Build history of the part. All positions in model axes, mm. A direction names the side the tool comes from. Give positions to 0.01 mm unless a question says otherwise; leave off trailing zeros. Order: outer loops, then holes, each group sorted by start corner. A loop starts at its lowest first (then second) coordinate and runs counter-clockwise, first axis right, second up. Notation, with made-up numbers: (-32, 23) -> (2, 23) arc R25 cw to (2, 59) -> close; hole circle Ø7 at (3.5, 29). An arc over 180 degrees is marked (long way). One line per question, with ' | ' between items. Start each with the question number.
(1) Drill centre lines: L1, parallel to X at y = 57.15, z = 11; L2, parallel to Y at x = 24, z = 18; L3, parallel to X at y = 52, z = 18.5. Where is each one in solid material? Low to high. Write a range as from..to.
(2) Pull direction Z, two halves, no side cores. Call faces 1 (the face through (5.02, 55.83, 9.66)), 2 (the face through (52.37, 74.27, 15.73)), 3 (the face through (35, 39, 2.54)): +Z half, -Z half, draft (parallel to the pull), parting line (faces both ways), or undercut.
(3) Which spindle directions (+Z, -Z, +X, -X, +Y, -Y) get a long thin tool onto all of the face, cutting with end or side? Do faces 4 (the face through (64.41, 68.15, 10.68)), 5 (the face through (35, 76.2, 9)). Say none if no direction does.
(4) Pin check, flat tips, straight feed: pin 1 Ø10 at (x, y) = (41, 9.5) entering from +Z; pin 2 Ø2 at (x, y) = (64.77, 57.15) entering from -Z. Stop position of each tip, or through.
(5) Cut at A-A (y = 38.1). Give the cut face in (x, z), then the cut area to 3 significant figures.
(6) Cut at B-B (x = 16). Give the cut face in (y, z), then the cut area to 3 significant figures.
(7) Cut at C-C (y = 71). Give the cut face in (x, z), then the cut area to 3 significant figures.
Autodesk Inventor part; units mm, degrees
ref_plane "YZ Plane" through (0, 0, 0) normal (1, 0, 0) x (0, 1, 0)
ref_plane "XZ Plane" through (0, 0, 0) normal (0, 1, 0) x (-1, 0, 0)
ref_plane "XY Plane" through (0, 0, 0) normal (0, 0, 1) x (1, 0, 0)
sketch "Sketch1" plane through (0, 0, 0) normal (0, 0, 1) x (1, 0, 0)
  line L0 (0, 0) -> (69.85, 0)
  line L1 (69.85, 0) -> (69.85, 76.2)
  line L2 (69.85, 76.2) -> (0, 76.2)
  line L3 (0, 76.2) -> (0, 0)
  line L4 (0, 76.2) -> (7.62, 76.2)
  line L5 (7.62, 3.81) -> (62.23, 3.81)
  line L6 (58.42, 72.39) -> (7.62, 72.39)
  line L7 (7.62, 72.39) -> (11.43, 72.39)
  line L8 (0, 76.2) -> (69.85, 76.2)
  line L9 (34.925, 76.2) -> (50.165, 76.2)
  line L10 (50.165, 76.2) -> (50.165, 69.1676)
  line L11 (34.925, 76.2) -> (19.685, 76.2)
  line L12 (19.685, 76.2) -> (14.9225, 76.2)
  line L13 (0, 76.2) -> (0, 57.15)
  line L14 (19.685, 76.2) -> (13.9303, 76.2)
  arc A0 (11.43, 72.39) -> (7.62, 60.96) centre (11.43, 66.04) ccw
  line L15 (7.62, 3.81) -> (11.43, 3.81)
  line L16 (11.43, 3.81) -> (11.43, 10.16)
  line L17 (62.23, 3.81) -> (58.42, 3.81)
  line L18 (58.42, 3.81) -> (58.42, 10.16)
  arc A1 (7.62, 15.24) -> (11.43, 3.81) centre (11.43, 10.16) ccw
  arc A2 (58.42, 3.81) -> (62.23, 15.24) centre (58.42, 10.16) ccw
  arc A3 (62.23, 60.96) -> (58.42, 72.39) centre (58.42, 66.04) ccw
  line L19 (62.23, 15.24) -> (62.23, 60.96)
  line L20 (7.62, 60.96) -> (7.62, 15.24)
  dimension "d9" = 7.62
  dimension "d13" = 15.24
  dimension "d18" = 19.05
  dimension "d24" = 6.35
  dimension "d25" = 3.81
  dimension "d26" = 6.35
extrude "Extrusion1" add sketch "Sketch1" along normal blind 19.05
sketch "Sketch3" plane through (0, 0, 0) normal (0, 0, -1) x (-1, 0, 0)
  arc A0 (-11.43, 3.81) -> (-7.62, 15.24) centre (-11.43, 10.16) ccw
  line L0 (-11.43, 3.81) -> (-58.42, 3.81)
  arc A1 (-62.23, 15.24) -> (-58.42, 3.81) centre (-58.42, 10.16) ccw
  line L1 (-62.23, 15.24) -> (-62.23, 60.96)
  arc A2 (-58.42, 72.39) -> (-62.23, 60.96) centre (-58.42, 66.04) ccw
  line L2 (-58.42, 72.39) -> (-11.43, 72.39)
  arc A3 (-7.62, 60.96) -> (-11.43, 72.39) centre (-11.43, 66.04) ccw
  line L3 (-7.62, 60.96) -> (-7.62, 15.24)
  line L4 (0, 76.2) -> (0, 0)
  line L5 (-69.85, 76.2) -> (0, 76.2)
  line L6 (-69.85, 0) -> (-69.85, 76.2)
  line L7 (0, 0) -> (-69.85, 0)
  line L8 (0, 76.2) -> (-5.08, 76.2)
  line L9 (-69.85, 76.2) -> (0, 76.2)
  line L10 (-5.08, 76.2) -> (-5.08, 0)
  line L11 (-5.08, 76.2) -> (-5.08, 57.15)
  line L12 (-5.08, 0) -> (-5.08, 19.05)
  line L13 (-69.85, 0) -> (-64.77, 0)
  line L14 (0, 0) -> (-69.85, 0)
  line L15 (-64.77, 0) -> (-64.77, 19.05)
  line L16 (-69.85, 76.2) -> (-64.77, 76.2)
  line L17 (-64.77, 76.2) -> (-64.77, 57.15)
  line L18 (-64.77, 57.15) -> (-64.77, 38.1)
  line L19 (-5.08, 57.15) -> (-5.08, 38.1)
  dimension "d31" = 5.08
  dimension "d32" = 19.05
  dimension "d33" = 19.05
  dimension "d34" = 5.08
  dimension "d35" = 19.05
  dimension "d36" = 5.08
  dimension "d37" = 19.05
  dimension "d38" = 19.05
  dimension "d39" = 19.05
hole "Hole1" at (64.77, 57.15, 0) at (64.77, 38.1, 0) at (64.77, 19.05, 0) at (5.08, 19.05, 0) at (5.08, 38.1, 0) at (5.08, 57.15, 0) direction (0, 0, 1) diameter 2.6416 depth 23.0124 tip angle 118
sketch "Sketch7" plane through (0, 0, 0) normal (0, 0, -1) x (-1, 0, 0)
  circle A0 centre (-5.08, 38.1) radius 1.3208
  circle A1 centre (-64.77, 19.05) radius 1.3208
  circle A2 centre (-64.77, 57.15) radius 1.3208
  circle A3 centre (-64.77, 38.1) radius 1.3208
  circle A4 centre (-5.08, 19.05) radius 1.3208
  circle A5 centre (-5.08, 57.15) radius 1.3208
  arc A6 (-11.43, 3.81) -> (-7.62, 15.24) centre (-11.43, 10.16) ccw
  line L0 (-11.43, 3.81) -> (-58.42, 3.81)
  arc A7 (-62.23, 15.24) -> (-58.42, 3.81) centre (-58.42, 10.16) ccw
  line L1 (-62.23, 15.24) -> (-62.23, 60.96)
  arc A8 (-58.42, 72.39) -> (-62.23, 60.96) centre (-58.42, 66.04) ccw
  line L2 (-58.42, 72.39) -> (-11.43, 72.39)
  arc A9 (-7.62, 60.96) -> (-11.43, 72.39) centre (-11.43, 66.04) ccw
  line L3 (-7.62, 60.96) -> (-7.62, 15.24)
  line L4 (0, 76.2) -> (0, 0)
  line L5 (-69.85, 76.2) -> (0, 76.2)
  line L6 (-69.85, 0) -> (-69.85, 76.2)
  line L7 (0, 0) -> (-69.85, 0)
extrude "Extrusion4" add sketch "Sketch7" against normal blind 2.54 contours L0 A7 L1 A8 L2 A9 L3 A6 | L4 L7 L6 L5
sketch "Sketch8" plane through (0, 76.2, 19.05) normal (0, 1, 0) x (1, 0, 0)
  point P0 (0, 19.05)
sketch "Sketch9" plane through (0, 76.2, 19.05) normal (0, 1, 0) x (1, 0, 0)
  line L0 (0, 19.05) -> (0, 0)
  line L1 (69.85, 0) -> (0, 0)
  line L2 (69.85, 19.05) -> (69.85, 0)
  line L3 (69.85, 19.05) -> (0, 19.05)
  line L4 (0, 19.05) -> (69.85, 19.05)
  line L5 (0, 19.05) -> (69.85, 19.05)
  line L6 (34.925, 19.05) -> (34.925, 8.636)
  line L7 (34.925, 8.636) -> (19.685, 8.636)
  dimension "d74" = 10.414
  dimension "d75" = 15.24
hole "Hole4" at (19.685, 76.2, 10.414) direction (0, -1, 0) diameter 9.525 depth 25.4 tip angle 118
sketch "Sketch10" plane through (0, 76.2, 19.05) normal (0, 1, 0) x (1, 0, 0)
  circle A0 centre (19.685, 8.636) radius 4.7625
  line L0 (0, 19.05) -> (0, 0)
  line L1 (69.85, 0) -> (0, 0)
  line L2 (69.85, 19.05) -> (69.85, 0)
  line L3 (69.85, 19.05) -> (0, 19.05)
  line L4 (69.85, 19.05) -> (0, 19.05)
  line L5 (69.85, 19.05) -> (0, 19.05)
  line L6 (34.925, 19.05) -> (34.925, 8.636)
  line L7 (34.925, 8.636) -> (50.165, 8.636)
  dimension "d83" = 15.24
  dimension "d91" = 10.414
hole "Hole5" at (50.165, 76.2, 10.414) direction (0, -1, 0) diameter 11.5094 depth 25.4 tip angle 118
sketch "Sketch11" plane through (0, 76.2, 19.05) normal (0, 1, 0) x (1, 0, 0)
  circle A0 centre (50.165, 8.636) radius 5.7547
  circle A1 centre (19.685, 8.636) radius 4.7625
  line L0 (0, 19.05) -> (0, 0)
  line L1 (69.85, 0) -> (0, 0)
  line L2 (69.85, 19.05) -> (69.85, 0)
  line L3 (69.85, 19.05) -> (0, 19.05)
properties part number "Light-tight_box"
Result set:
1) L1: x = 0..3.76, 6.4..7.62, 62.23..63.45, 66.09..69.85 | L2: y = 0..3.81, 72.39..76.2 | L3: x = 0..7.62, 62.23..69.85
2) face 1: draft | face 2: undercut | face 3: +Z half
3) face 4: +Z | face 5: +Z, -Z, +X, -X, +Y
4) pin 1: stops at z = 2.54 | pin 2: passes through
5) outline: (0, 0) -> (3.76, 0) -> (3.76, 19.05) -> (0, 19.05) -> close; (6.4, 0) -> (63.45, 0) -> (63.45, 19.05) -> (62.23, 19.05) -> (62.23, 2.54) -> (7.62, 2.54) -> (7.62, 19.05) -> (6.4, 19.05) -> close; (66.09, 0) -> (69.85, 0) -> (69.85, 19.05) -> (66.09, 19.05) -> close | area: 328 mm2
6) outline: (0, 0) -> (76.2, 0) -> (76.2, 7.4) -> (72.39, 7.4) -> (72.39, 2.54) -> (3.81, 2.54) -> (3.81, 19.05) -> (0, 19.05) -> close; (72.39, 13.43) -> (76.2, 13.43) -> (76.2, 19.05) -> (72.39, 19.05) -> close | area: 296 mm2
7) outline: (0, 0) -> (69.85, 0) -> (69.85, 19.05) -> (62.38, 19.05) -> (62.38, 2.54) -> (7.47, 2.54) -> (7.47, 19.05) -> (0, 19.05) -> close | area: 424 mm2
